from build123d import *

# Parameters (mm, degrees)
SKETCH1_W           = 204
SKETCH1_H           = 80
BOSS_EXTRUDE1_DEPTH = 8
SKETCH2_W           = 204
SKETCH2_H           = 70
CUT_EXTRUDE1_DEPTH  = 3
SKETCH3_R           = 5
CUT_EXTRUDE2_DEPTH  = 3
SKETCH4_R           = 2.5
CUT_EXTRUDE3_DEPTH  = 3
CHAMFER1_SIZE       = 3
CHAMFER2_SIZE       = 0.25


with BuildPart() as part:
    # Sketch1 → Boss-Extrude1 (new body)
    with BuildSketch(Plane(origin=(0, 0, 0), x_dir=(1, 0, 0), z_dir=(0, 1, 0))):
        with Locations((102, 40)):
            Rectangle(SKETCH1_W, SKETCH1_H)
    extrude(amount=BOSS_EXTRUDE1_DEPTH)

    # Sketch2 → Cut-Extrude1 (cut)
    with BuildSketch(Plane(origin=(0, 8, 0), x_dir=(1, 0, 0), z_dir=(0, 1, 0))):
        with Locations((102, 40)):
            Rectangle(SKETCH2_W, SKETCH2_H)
    extrude(amount=-CUT_EXTRUDE1_DEPTH, mode=Mode.SUBTRACT)

    # Sketch3 → Cut-Extrude2 (cut)
    with BuildSketch(Plane(origin=(0, 5, 0), x_dir=(1, 0, 0), z_dir=(0, 1, 0))):
        with Locations((31.247103349, 61.25)):
            Circle(SKETCH3_R)
        with Locations((95.247103349, 61.25)):
            Circle(SKETCH3_R)
        with Locations((31.247103349, 18.75)):
            Circle(SKETCH3_R)
        with Locations((95.247103349, 18.75)):
            Circle(SKETCH3_R)
    extrude(amount=-CUT_EXTRUDE2_DEPTH, mode=Mode.SUBTRACT)

    # Sketch4 → Cut-Extrude3 (cut, through all)
    with BuildSketch(Plane(origin=(0, 2, 0), x_dir=(1, 0, 0), z_dir=(0, 1, 0))):
        with Locations((31.247103349, 61.25)):
            Circle(SKETCH4_R)
        with Locations((95.247103349, 61.25)):
            Circle(SKETCH4_R)
        with Locations((95.247103349, 18.75)):
            Circle(SKETCH4_R)
        with Locations((31.247103349, 18.75)):
            Circle(SKETCH4_R)
    extrude(amount=-CUT_EXTRUDE3_DEPTH, mode=Mode.SUBTRACT)

    # Chamfer1
    chamfer1_edges = [part.edges().sort_by_distance(p)[0] for p in [
        (204, 4, -80),
        (204, 4, 0),
    ]]
    chamfer(chamfer1_edges, length=CHAMFER1_SIZE)

    # Chamfer2
    chamfer2_edges = [part.edges().sort_by_distance(p)[0] for p in [
        (102, 8, -5),
        (102, 8, -75),
        (100.5, 8, -80),
        (100.5, 8, 0),
    ]]
    chamfer(chamfer2_edges, length=CHAMFER2_SIZE)


solid = part.part
Verification items for the finished model (mm, model axes). A direction names the side the tool comes from. Coordinates: 2 decimals unless noted, no trailing zeros. Order: outer loops, then holes, each group sorted by start corner. A loop starts at its lowest first (then second) coordinate and runs counter-clockwise, first axis right, second up. Notation, with made-up numbers: M 0.25,33 L 59.25,33 A17 ccw 59.25,50 Z; hole C -25.5,-9.75 d7. An arc over 180 degrees is marked long. One line per item, written item: value. Start each with the question number.
Item 1: Sectioned sample at D-D (z = -52). Enter the section's corners in (x, y), then the cut area to 3 significant figures.
Item 2: Sectioned sample at A-A (z = -61.25). Enter the section's corners in (x, y).
Item 3: Scan lines: probe 1 along X at (y, z) = (0.9, -18.75); probe 2 along X at (y, z) = (3.5, -20.5); probe 3 along Z at (x, y) = (162, 5.5). Record each from-to range of solid material in increasing order.
Item 4: Mould release check, pull along Z, two halves, no side actions. Record for faces 4 (the flat face through (101, 0, -41)), 5 (the flat face through (99, 4, -80)), 6 (the cylindrical face through (33.556, 1.014, -60.292)), 7 (the cylindrical face through (32.59, 1.01, -20.86)): released by +Z, released by -Z, zero draft, split by the parting line, or undercut.
Item 5: Gauge pin test, flat ends, axial feed: pin 1 (3 mm diameter, centred on x = 95.25, z = -18.75, fed in from +Y); pin 2 (6 mm diameter, centred on x = 72, z = -11, fed in from +Y); pin 3 (5 mm diameter, centred on x = 93, z = -61, fed in from +Y). Record the tip position at first contact, or that the pin passes through.
Item 6: Sectioned sample at C-C (x = 179). Enter the section's corners in (y, z).
Item 7: Sectioned sample at B-B (y = 3.25). Enter the section's corners in (x, z), then the cut area to 3 significant figures.
Item 8: Access from +Z, -Z, +X, -X, +Y, -Y to the whole of each face (thin tool, end or side, straight path). Record for faces 1 (the flat face through (101, 5, -40)), 2 (the flat face through (99, 4, 0)), 3 (the flat face through (97.4, 2, -16.6)).
Conclusion:
1. outline: M 0,0 L 204,0 L 204,5 L 0,5 Z
1. area: 1,020 mm^2
2. outline: M 0,0 L 28.75,0 L 28.75,2 L 26.25,2 L 26.25,5 L 0,5 Z; M 33.75,0 L 92.75,0 L 92.75,2 L 90.25,2 L 90.25,5 L 36.25,5 L 36.25,2 L 33.75,2 Z; M 97.75,0 L 204,0 L 204,5 L 100.25,5 L 100.25,2 L 97.75,2 Z
3. probe 1: x = 0 to 28.75, 33.75 to 92.75, 97.75 to 204
3. probe 2: x = 0 to 26.56, 35.93 to 90.56, 99.93 to 204
3. probe 3: z = -80 to -75, -5 to 0
4. face 4: zero draft
4. face 5: released by -Z
4. face 6: undercut
4. face 7: undercut
5. pin 1: passes through
5. pin 2: stops at y = 5
5. pin 3: stops at y = 2
6. outline: M 0,-80 L 7.75,-80 L 8,-79.75 L 8,-75.25 L 7.75,-75 L 5,-75 L 5,-5 L 7.75,-5 L 8,-4.75 L 8,-0.25 L 7.75,0 L 0,0 Z
7. outline: M 0,-80 L 201,-80 L 204,-77 L 204,-3 L 201,0 L 0,0 Z; hole C 31.25,-61.25 d10; hole C 31.25,-18.75 d10; hole C 95.25,-61.25 d10; hole C 95.25,-18.75 d10
7. area: 16,000 mm^2
8. face 1: +X, -X, +Y
8. face 2: +Z, +X, -X, +Y, -Y
8. face 3: +Y
